Work out the finished part from the listing and answer in its coordinate system (mm). Face numbers are marked on the shaded views. Give positions to 0.01 mm unless a question says otherwise; leave off trailing zeros. Write each loop counter-clockwise with the first axis right and the second up, starting at its lowest first coordinate (ties: lowest second). Pieces come first, ordered by that corner, then holes.
1) Find section D-D (y = 4.5). Count the separate pieces of the cut face and the enclosed holes in it, plus the area to 3 significant figures.
2) Determine the mould class of the marked faces 1, 2 and 3 for opening direction Z: pulls with the +Z half, pulls with the -Z half, needs draft (parallel to the pull), parting line crosses it, or undercut.
3) Find section B-B (z = 2.5). Determine the outline of the cut face in (x, y).
4) Straight lines are drawn through the part: probe 1 along X at (y, z) = (1.5, -15.5); probe 2 along X at (y, z) = (4.6, 2); probe 3 along X at (y, z) = (4.35, 7). For each, find the intervals that lie inside material, in ascending order.
5) Find section C-C (z = -21). Determine the outline of the cut face in (x, y), plus the area to 3 significant figures.
6) Find section A-A (x = 0). Determine the outline of the cut face in (y, z).
7) Given pin 1 Ø3 at (x, z) = (6.5, 6) entering from -Y, flat-ended and moving along its own axis, determine where the tip first touches the part or whether it passes through.
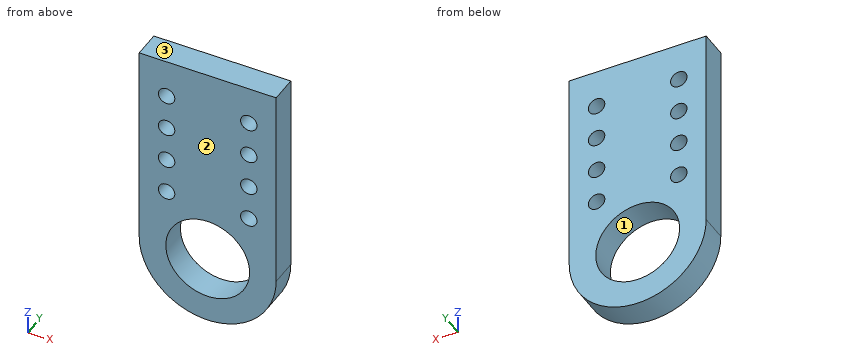
```python
from build123d import *

# Parameters (mm, degrees)
SKETCH_1_R      = 7.65
SKETCH_1_R_2    = 1.5
EXTRUDE_1_DEPTH = 5


with BuildPart() as part:
    # Эскиз1 → Бобышка-Вытянуть1 (new body)
    with BuildSketch(Plane(origin=(0, 0, 0), x_dir=(1, 0, 0), z_dir=(0, 1, 0))):
        with BuildLine():
            Line((-12.5, 15.852233677), (-12.5, -21.647766323))
            Line((-12.5, -21.647766323), (12.5, -21.647766323))
            Line((12.5, -21.647766323), (12.5, 15.852233677))
            ThreePointArc((12.5, 15.852233677), (0, 28.352233677), (-12.5, 15.852233677))
        make_face()
        with Locations((0, 15.852233677)):
            Circle(SKETCH_1_R, mode=Mode.SUBTRACT)
        with Locations((-7.5, -14.647766323)):
            Circle(SKETCH_1_R_2, mode=Mode.SUBTRACT)
        with Locations((7.5, -14.647766323)):
            Circle(SKETCH_1_R_2, mode=Mode.SUBTRACT)
        with Locations((-7.5, -8.147766323)):
            Circle(SKETCH_1_R_2, mode=Mode.SUBTRACT)
        with Locations((7.5, -8.147766323)):
            Circle(SKETCH_1_R_2, mode=Mode.SUBTRACT)
        with Locations((-7.5, -1.647766323)):
            Circle(SKETCH_1_R_2, mode=Mode.SUBTRACT)
        with Locations((7.5, -1.647766323)):
            Circle(SKETCH_1_R_2, mode=Mode.SUBTRACT)
        with Locations((-7.5, 4.852233677)):
            Circle(SKETCH_1_R_2, mode=Mode.SUBTRACT)
        with Locations((7.5, 4.852233677)):
            Circle(SKETCH_1_R_2, mode=Mode.SUBTRACT)
    extrude(amount=EXTRUDE_1_DEPTH)


solid = part.part
```
Results:
1. separate pieces: 1
1. enclosed holes: 9
1. area: 943 mm2
2. face 1: undercut
2. face 2: needs draft
2. face 3: pulls with the +Z half
3. outline: (-12.5, 0) - (-8.73, 0) - (-8.73, 5) - (-12.5, 5) - close; (-6.27, 0) - (6.27, 0) - (6.27, 5) - (-6.27, 5) - close; (8.73, 0) - (12.5, 0) - (12.5, 5) - (8.73, 5) - close
4. probe 1: x = -12.5 to -7.64, 7.64 to 12.5
4. probe 2: x = -12.5 to -8.96, -6.04 to 6.04, 8.96 to 12.5
4. probe 3: x = -12.5 to -8.47, -6.53 to 6.53, 8.47 to 12.5
5. outline: (-11.39, 0) - (-5.66, 0) - (-5.66, 5) - (-11.39, 5) - close; (5.66, 0) - (11.39, 0) - (11.39, 5) - (5.66, 5) - close
5. area: 57.3 mm2
6. outline: (0, -28.35) - (5, -28.35) - (5, -23.5) - (0, -23.5) - close; (0, -8.2) - (5, -8.2) - (5, 21.65) - (0, 21.65) - close
7. pin 1: stops at y = 0
